Source: CAD feature listing. Evaluate the final solid. Frame: model axes, mm. A direction names the side the tool comes from. Coordinates: 2 decimals unless noted, no trailing zeros. Write each loop counter-clockwise with the first axis right and the second up, starting at its lowest first coordinate (ties: lowest second). Pieces come first, ordered by that corner, then holes. Notation, with made-up numbers: (30, 88) - (57, 88) arc R22 ccw to (57, 119) - close; hole circle Ø6 at (80, 35). An arc over 180 degrees is marked (long way). One line per question, with ' | ' between items.
from build123d import *

# Parameters (mm, degrees)
BOSS_EXTRUDE1_DEPTH = 20
SKETCH3_W           = 8
SKETCH3_H           = 8
CUT_EXTRUDE1_DEPTH  = 10
SKETCH4_R           = 1
CUT_EXTRUDE2_DEPTH  = 10
SKETCH5_W           = 4
SKETCH5_H           = 20
CUT_EXTRUDE3_DEPTH  = 0.5
SKETCH6_W           = 8
SKETCH6_H           = 3
BOSS_EXTRUDE2_DEPTH = 8
SKETCH4_2_R         = 1
BOSS_EXTRUDE3_DEPTH = 3
SKETCH7_W           = 20
SKETCH7_H           = 3
BOSS_EXTRUDE4_DEPTH = 3
SKETCH8_W           = 21.136904569
SKETCH8_H           = 7.074304785
CUT_EXTRUDE4_DEPTH  = 3
SKETCH9_R           = 0.85
CUT_EXTRUDE6_DEPTH  = 3
FILLET1_R           = 8
SKETCH9_5_R         = 0.85
CUT_EXTRUDE8_DEPTH  = 3
SKETCH10_W          = 22.706583138
SKETCH10_H          = 8.880510261
CUT_EXTRUDE9_DEPTH  = 0.85
SKETCH4_3_R         = 1
BOSS_EXTRUDE6_DEPTH = 3


with BuildPart() as part:
    # Sketch1 → Boss-Extrude1 (new body)
    with BuildSketch(Plane.XY):
        Polygon((0, 0), (0, 3), (4, 3), (7.927272727, 3), (7.927272727, 0), (15.927272727, 0), (15.927272727, -3), (7.927272727, -3), (4, -3), (4, 0), align=None)
    extrude(amount=BOSS_EXTRUDE1_DEPTH)

    # Sketch3 → Cut-Extrude1 (cut)
    with BuildSketch(Plane(origin=(0, 0, 0), x_dir=(1, 0, 0), z_dir=(0, 1, 0))):
        with Locations((11.927272727, -16)):
            Rectangle(SKETCH3_W, SKETCH3_H)
    extrude(amount=-CUT_EXTRUDE1_DEPTH, mode=Mode.SUBTRACT)

    # Sketch4 → Cut-Extrude2 (cut)
    with BuildSketch(Plane(origin=(0, 0, 0), x_dir=(1, 0, 0), z_dir=(0, 1, 0))):
        with Locations(Location((11.93972935, -3, 0), (0, 0, 270))):
            Circle(SKETCH4_R)
        with Locations(Location((11.93972935, -9, 0), (0, 0, 270))):
            Circle(SKETCH4_R)
    extrude(amount=-CUT_EXTRUDE2_DEPTH, mode=Mode.SUBTRACT)

    # Sketch5 → Cut-Extrude3 (cut)
    with BuildSketch(Plane.XZ):
        with Locations((2, 10)):
            Rectangle(SKETCH5_W, SKETCH5_H)
    extrude(amount=-CUT_EXTRUDE3_DEPTH, mode=Mode.SUBTRACT)

    # Sketch6 → Boss-Extrude2 (add)
    with BuildSketch(Plane.XY.offset(12)):
        with Locations((11.927272727, -1.5)):
            Rectangle(SKETCH6_W, SKETCH6_H)
    extrude(amount=BOSS_EXTRUDE2_DEPTH)

    # Sketch4_2 → Boss-Extrude3 (add)
    with BuildSketch(Plane(origin=(0, 0, 0), x_dir=(1, 0, 0), z_dir=(0, 1, 0))):
        with Locations((11.93972935, -9)):
            Circle(SKETCH4_2_R)
    extrude(amount=-BOSS_EXTRUDE3_DEPTH)

    # Sketch7 → Boss-Extrude4 (add)
    with BuildSketch(Plane(origin=(15.927272727, 0, 0), x_dir=(0, 0, -1), z_dir=(1, 0, 0))):
        with Locations((-10, -1.5)):
            Rectangle(SKETCH7_W, SKETCH7_H)
    extrude(amount=BOSS_EXTRUDE4_DEPTH)

    # Sketch8 → Cut-Extrude4 (cut)
    with BuildSketch(Plane.XY.offset(20)):
        with Locations((9.151850895, 0.075258561)):
            Rectangle(SKETCH8_W, SKETCH8_H)
    extrude(amount=-CUT_EXTRUDE4_DEPTH, mode=Mode.SUBTRACT)

    # Sketch9 → Cut-Extrude6 (cut)
    with BuildSketch(Plane(origin=(0, 0, 0), x_dir=(1, 0, 0), z_dir=(0, 1, 0))):
        with Locations(Location((10.063554841, -13.873545982, 0), (0, 0, 270))):
            Circle(SKETCH9_R)
    extrude(amount=-CUT_EXTRUDE6_DEPTH, mode=Mode.SUBTRACT)

    # Fillet1
    fillet1_edges = [part.edges().sort_by_distance(p)[0] for p in [
        (18.927272727, -1.5, 17),
    ]]
    fillet(fillet1_edges, radius=FILLET1_R)

    # Sketch9_5 → Cut-Extrude8 (cut)
    with BuildSketch(Plane(origin=(0, 0, 0), x_dir=(1, 0, 0), z_dir=(0, 1, 0))):
        with Locations(Location((10.063554841, -13.873545982, 0), (0, 0, 270))):
            Circle(SKETCH9_5_R)
        with Locations(Location((15.93972935, -3, 0), (0, 0, 270))):
            Circle(SKETCH9_5_R)
        with Locations(Location((16.217987441, -8.5, 0), (0, 0, 270))):
            Circle(SKETCH9_5_R)
        with Locations(Location((10.063554841, -3, 0), (0, 0, 270))):
            Circle(SKETCH9_5_R)
    extrude(amount=-CUT_EXTRUDE8_DEPTH, mode=Mode.SUBTRACT)

    # Sketch10 → Cut-Extrude9 (cut)
    with BuildSketch(Plane(origin=(0, 0, 0), x_dir=(-1, 0, 0), z_dir=(0, 0, -1))):
        with Locations((-10.194719533, 0.225775684)):
            Rectangle(SKETCH10_W, SKETCH10_H)
    extrude(amount=-CUT_EXTRUDE9_DEPTH, mode=Mode.SUBTRACT)

    # Sketch4_3 → Boss-Extrude6 (add)
    with BuildSketch(Plane(origin=(0, 0, 0), x_dir=(1, 0, 0), z_dir=(0, 1, 0))):
        with Locations((11.93972935, -3)):
            Circle(SKETCH4_3_R)
    extrude(amount=-BOSS_EXTRUDE6_DEPTH)


solid = part.part
Item 1: Ray query, line 1 along X through (y, z) = (-0.85, 3); line 2 along X through (y, z) = (-1.3, 8.5); line 3 along Y through (x, z) = (12.75, 5.25). Return the intervals inside material, ascending. Write a range as [from, to].
Check sheet entries:
line 1: [4, 9.21], [10.91, 15.09], [16.79, 18.93] | line 2: [4, 15.37], [17.07, 18.93] | line 3: [-3, 0]
Item 2: Cut plane C-C on y = -2.55. Return loops of the section in (x, z), and give its area (3 significant figures).
Check sheet entries:
outline: (4, 0.85) - (18.93, 0.85) - (18.93, 9) arc R8 ccw to (10.93, 17) - (4, 17) - close; hole circle Ø1.7 at (10.06, 3); hole circle Ø1.7 at (10.06, 13.87); hole circle Ø1.7 at (15.94, 3); hole circle Ø1.7 at (16.22, 8.5) | area: 218 mm²
Item 3: Cut plane A-A on z = 8.5. Return loops of the section in (x, y).
Check sheet entries:
outline: (0, 0.5) - (4, 0.5) - (4, -3) - (15.37, -3) - (15.37, 0) - (7.93, 0) - (7.93, 3) - (0, 3) - close; (17.07, -3) - (18.93, -3) - (18.93, 0) - (17.07, 0) - close
Item 4: Cut plane B-B on z = 3. Return loops of the section in (x, y), and give its area (3 significant figures).
Check sheet entries:
outline: (0, 0.5) - (4, 0.5) - (4, -3) - (9.21, -3) - (9.21, 0) - (7.93, 0) - (7.93, 3) - (0, 3) - close; (10.91, -3) - (15.09, -3) - (15.09, 0) - (10.91, 0) - close; (16.79, -3) - (18.93, -3) - (18.93, 0) - (16.79, 0) - close | area: 56.4 mm²
Item 5: Cut plane D-D on x = 3.5. Return loops of the section in (y, z).
Check sheet entries:
outline: (0.5, 0.85) - (3, 0.85) - (3, 17) - (0.5, 17) - close
Item 6: Mould query, pull axis X, two halves, no side actions, for faces 1 (the face through (13, 0, 9)), 2 (the face through (16.935, -1.479, 8.957)), 3 (the face through (7.927, 2, 9)). Classes: pulls with the +X half, pulls with the -X half, needs draft (parallel to the pull), parting line crosses it, or undercut.
Check sheet entries:
face 1: needs draft | face 2: undercut | face 3: pulls with the +X half
Item 7: Access query for faces 4 (the face through (4, -1, 9)), 5 (the face through (10, -1, 0.85)). Directions: +Z, -Z, +X, -X, +Y, -Y. A direction counts if a zero-diameter tool reaches every point of the face in a straight line with its end or side. Return the directions, or none.
Check sheet entries:
face 4: +Z, -Z, -X, -Y | face 5: -Z, +X, -X, +Y, -Y
Item 8: Pin query (flat end, axial travel): pin 1 Ø2.5 at (x, z) = (16.22, 8.5) entering from +Y; pin 2 Ø3 at (y, z) = (-1.5, 7.5) entering from -X. Return the tip coordinate at first contact, or that it passes through.
Check sheet entries:
pin 1: y = 0 | pin 2: x = 4
